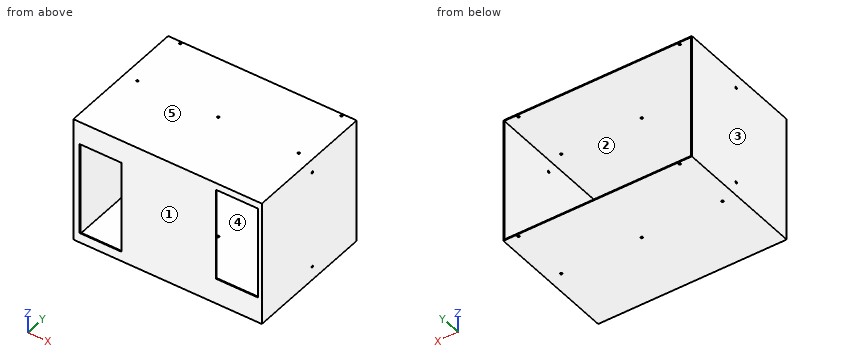
from build123d import *

# Parameters (mm, degrees)
CROQUIS1_W                 = 270
CROQUIS1_H                 = 190
SALIENTE_EXTRUIR1_DEPTH    = 90
CROQUIS2_W                 = 60
CROQUIS2_H                 = 133
CORTAR_EXTRUIR2_DEPTH      = 35.7
CROQUIS6_W                 = 267.2
CROQUIS6_H                 = 177.2
CORTAR_EXTRUIR3_DEPTH      = 188.6
CROQUIS8_R                 = 1.5
CORTAR_EXTRUIR4_DEPTH      = 300
CORTAR_EXTRUIR6_DEPTH      = 135
CORTAR_EXTRUIR6_DEPTH_BACK = 368
CROQUIS10_R                = 1.5
CORTAR_EXTRUIR7_DEPTH      = 112
CORTAR_EXTRUIR7_DEPTH_BACK = 260.1
CROQUIS11_R                = 1.5


with BuildPart() as part:
    # Croquis1 → Saliente-Extruir1 (new, symmetric)
    with BuildSketch(Plane.XY):
        with Locations((0, 48.4)):
            Rectangle(CROQUIS1_W, CROQUIS1_H)
    extrude(amount=SALIENTE_EXTRUIR1_DEPTH, both=True)

    # Croquis2 → Cortar-Extruir2 (cut, symmetric)
    with BuildSketch(Plane(origin=(0, -46.6, 0), x_dir=(1, 0, 0), z_dir=(0, 1, 0))):
        with Locations((-96, 9.5)):
            Rectangle(CROQUIS2_W, CROQUIS2_H)
        with Locations((99.26, -13.5)):
            Rectangle(CROQUIS2_W, CROQUIS2_H)
    extrude(amount=CORTAR_EXTRUIR2_DEPTH, both=True, mode=Mode.SUBTRACT)

    # Croquis6 → Cortar-Extruir3 (cut)
    with BuildSketch(Plane(origin=(0, 143.4, 0), x_dir=(1, 0, 0), z_dir=(0, 1, 0))):
        Rectangle(CROQUIS6_W, CROQUIS6_H)
    extrude(amount=-CORTAR_EXTRUIR3_DEPTH, mode=Mode.SUBTRACT)

    # Croquis8 → Cortar-Extruir4 (cut, symmetric)
    with BuildSketch(Plane.XY.offset(90)):
        with Locations((-115.475, 54.65)):
            Circle(CROQUIS8_R)
        with Locations((0, 54.65)):
            Circle(CROQUIS8_R)
        with Locations((115.475, 54.65)):
            Circle(CROQUIS8_R)
    extrude(amount=CORTAR_EXTRUIR4_DEPTH, both=True, mode=Mode.SUBTRACT)

    # Croquis10 → Cortar-Extruir6 (cut, two sides: drawn at the far end of the back side and taken through both)
    with BuildSketch(Plane.ZY.offset(135).offset(-CORTAR_EXTRUIR6_DEPTH_BACK)):
        with Locations(Location((-70.475, 54.65, 0), (0, 0, 180))):
            Circle(CROQUIS10_R)
        with Locations(Location((70.475, 54.65, 0), (0, 0, 180))):
            Circle(CROQUIS10_R)
    extrude(amount=CORTAR_EXTRUIR6_DEPTH + CORTAR_EXTRUIR6_DEPTH_BACK, mode=Mode.SUBTRACT)

    # Croquis11 → Cortar-Extruir7 (cut, two sides: drawn at the far end of the back side and taken through both)
    with BuildSketch(Plane.XY.offset(90).offset(-CORTAR_EXTRUIR7_DEPTH_BACK)):
        with Locations(Location((-115.475, 140.275, 0), (0, 0, 180))):
            Circle(CROQUIS11_R)
        with Locations(Location((115.475, 140.275, 0), (0, 0, 180))):
            Circle(CROQUIS11_R)
    extrude(amount=CORTAR_EXTRUIR7_DEPTH + CORTAR_EXTRUIR7_DEPTH_BACK, mode=Mode.SUBTRACT)


solid = part.part
Geometry check sheet. Reference: the model listing, model coordinates, mm. Face numbers are marked on the shaded views. A direction names the side the tool comes from. Round coordinates to 2 decimals unless told otherwise and drop trailing zeros. Order: outer loops, then holes, each group sorted by start corner. A loop starts at its lowest first (then second) coordinate and runs counter-clockwise, first axis right, second up. Notation, with made-up numbers: (-30, 59) - (-9, 59) arc R22 cw to (-9, 74) - close; hole circle Ø7 at (16, 42). An arc over 180 degrees is marked (long way). One line per question, with ' | ' between items. Start each with the question number.
(1) Access from +Z, -Z, +X, -X, +Y, -Y to the whole of each face (thin tool, end or side, straight path). Record for the marked faces 4 and 5.
(2) Thickness scan on L1, parallel to Z at x = 109.5, y = 114; L2, parallel to X at y = 3.5, z = 35.5; L3, parallel to Y at x = 0, z = 89. Record the ranges inside material, lowest first. Write a range as [from, to].
(3) Depth check by flat-ended pin: pin 1 Ø1.8 at (x, y) = (-115.475, 140.275) entering from -Z; pin 2 Ø5 at (x, z) = (59.5, 37.5) entering from +Y. Enter the tip coordinate at first touch or a pass-through.
(4) Sectioned sample at A-A on z = 20. Record the cut outline in (x, y).
(5) Sectioned sample at C-C on y = -22.5. Record the cut outline in (x, z).
(6) Sectioned sample at B-B on x = -69.5. Record the cut outline in (y, z).
(7) Sectioned sample at D-D on x = -32.5. Record the cut outline in (y, z).
(8) Release check for a two-part mould opening along X. For the marked faces 1, 2 and 3 record: released by +X, released by -X, zero draft, split by the parting line, or undercut.
Conclusion:
1) face 4: +Y | face 5: +Z, +X, -X, +Y, -Y
2) L1: z = [-90, -88.6], [88.6, 90] | L2: x = [-135, -133.6], [133.6, 135] | L3: y = [-46.6, 53.15], [56.15, 143.4]
3) pin 1: passes through | pin 2: stops at y = -45.2
4) outline: (-135, -46.6) - (-126, -46.6) - (-126, -45.2) - (-133.6, -45.2) - (-133.6, 143.4) - (-135, 143.4) - close; (-66, -46.6) - (69.26, -46.6) - (69.26, -45.2) - (-66, -45.2) - close; (129.26, -46.6) - (135, -46.6) - (135, 143.4) - (133.6, 143.4) - (133.6, -45.2) - (129.26, -45.2) - close
5) outline: (-135, -90) - (135, -90) - (135, 90) - (-135, 90) - close; hole (-133.6, -88.6) - (133.6, -88.6) - (133.6, 88.6) - (-133.6, 88.6) - close
6) outline: (-46.6, -90) - (143.4, -90) - (143.4, -88.6) - (-45.2, -88.6) - (-45.2, -76) - (-46.6, -76) - close; (-46.6, 57) - (-45.2, 57) - (-45.2, 88.6) - (143.4, 88.6) - (143.4, 90) - (-46.6, 90) - close
7) outline: (-46.6, -90) - (143.4, -90) - (143.4, -88.6) - (-45.2, -88.6) - (-45.2, 88.6) - (143.4, 88.6) - (143.4, 90) - (-46.6, 90) - close
8) face 1: zero draft | face 2: undercut | face 3: released by -X
